Geometry: final body of the model. Coordinates: model frame, mm. Coordinates: 2 decimals unless noted, no trailing zeros. Loops run counter-clockwise (first coordinate to the right, second up) from the corner with the lowest first, then second, coordinate; pieces in that order, holes last. Notation, with made-up numbers: (-12.75, -18.75) -> (18.25, -18.75) arc R34 cw to (18.25, 13.25) -> close; hole circle Ø5 at (70.25, 2.25). An arc over 180 degrees is marked (long way). One line per item, written item: value. Start each with the question number.
from build123d import *

# Parameters (mm, degrees)
SKETCH1_W           = 70
SKETCH1_H           = 70
SKETCH1_R           = 5.8
SKETCH1_R_2         = 4.6
SKETCH1_R_3         = 2
BOSS_EXTRUDE1_DEPTH = 5
FILLET1_R           = 2
FILLET2_R           = 2


with BuildPart() as part:
    # Sketch1 → Boss-Extrude1 (new body)
    with BuildSketch(Plane.XY):
        Rectangle(SKETCH1_W, SKETCH1_H)
        with Locations((-27, 27)):
            Circle(SKETCH1_R, mode=Mode.SUBTRACT)
        with Locations((27, 27)):
            Circle(SKETCH1_R, mode=Mode.SUBTRACT)
        with Locations((27, -27)):
            Circle(SKETCH1_R, mode=Mode.SUBTRACT)
        with Locations((-27, -27)):
            Circle(SKETCH1_R, mode=Mode.SUBTRACT)
        Circle(SKETCH1_R_2, mode=Mode.SUBTRACT)
        with Locations((0, 27)):
            Circle(SKETCH1_R_3, mode=Mode.SUBTRACT)
        with Locations((0, -27)):
            Circle(SKETCH1_R_3, mode=Mode.SUBTRACT)
    extrude(amount=BOSS_EXTRUDE1_DEPTH)

    # Fillet1
    fillet1_edges = [part.edges().sort_by_distance(p)[0] for p in [
        (-35, 35, 2.5),
        (35, 35, 2.5),
        (35, -35, 2.5),
    ]]
    fillet(fillet1_edges, radius=FILLET1_R)

    # Fillet2
    fillet2_edges = [part.edges().sort_by_distance(p)[0] for p in [
        (-35, -35, 2.5),
    ]]
    fillet(fillet2_edges, radius=FILLET2_R)


solid = part.part
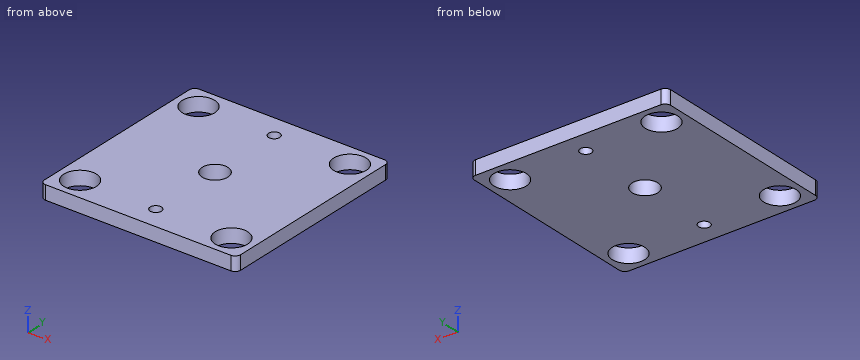
1. Line query: L1, parallel to Y at x = 27, z = 2.35; L2, parallel to Y at x = 0, z = 3.45; L3, parallel to Y at x = -23, z = 2.4. Output: solid intervals per line, ascending. Write a range as [from, to].
2. Section B-B on y = -27. Return the cut outline in (x, z).
3. Pin query (flat end, axial travel): pin 1 Ø7 at (x, y) = (-27, -27) entering from +Z. Return the tip coordinate at first contact, or that it passes through.
4. Section C-C on z = 3.35. Return the cut outline in (x, y), plus the area to 3 significant figures.
5. Section A-A on x = 27. Return the cut outline in (y, z), plus the area to 3 significant figures.
6. Section D-D on x = 0. Return the cut outline in (y, z), plus the area to 3 significant figures.
Checks:
1. L1: [-35, -32.8], [-21.2, 21.2], [32.8, 35]
1. L2: [-35, -29], [-25, -4.6], [4.6, 25], [29, 35]
1. L3: [-35, -31.2], [-22.8, 22.8], [31.2, 35]
2. outline: (-35, 0) -> (-32.8, 0) -> (-32.8, 5) -> (-35, 5) -> close; (-21.2, 0) -> (-2, 0) -> (-2, 5) -> (-21.2, 5) -> close; (2, 0) -> (21.2, 0) -> (21.2, 5) -> (2, 5) -> close; (32.8, 0) -> (35, 0) -> (35, 5) -> (32.8, 5) -> close
3. pin 1: through
4. outline: (-35, -33) arc R2 ccw to (-33, -35) -> (33, -35) arc R2 ccw to (35, -33) -> (35, 33) arc R2 ccw to (33, 35) -> (-33, 35) arc R2 ccw to (-35, 33) -> close; hole circle Ø11.6 at (-27, -27); hole circle Ø11.6 at (-27, 27); hole circle Ø9.2 at (0, 0); hole circle Ø4 at (0, -27); hole circle Ø4 at (0, 27); hole circle Ø11.6 at (27, -27); hole circle Ø11.6 at (27, 27)
4. area: 4,380 mm²
5. outline: (-35, 0) -> (-32.8, 0) -> (-32.8, 5) -> (-35, 5) -> close; (-21.2, 0) -> (21.2, 0) -> (21.2, 5) -> (-21.2, 5) -> close; (32.8, 0) -> (35, 0) -> (35, 5) -> (32.8, 5) -> close
5. area: 234 mm²
6. outline: (-35, 0) -> (-29, 0) -> (-29, 5) -> (-35, 5) -> close; (-25, 0) -> (-4.6, 0) -> (-4.6, 5) -> (-25, 5) -> close; (4.6, 0) -> (25, 0) -> (25, 5) -> (4.6, 5) -> close; (29, 0) -> (35, 0) -> (35, 5) -> (29, 5) -> close
6. area: 264 mm²
